Can you work these out from the model? Positions are in its coordinate system, mm. A direction names the side the tool comes from. Coordinates: 2 decimals unless noted, no trailing zeros. Order: outer loops, then holes, each group sorted by start corner. A loop starts at its lowest first (then second) coordinate and runs counter-clockwise, first axis right, second up. Notation, with made-up numbers: (14, 32.5) -> (37, 32.5) arc R18 ccw to (37, 60.5) -> close; hole circle Ø6 at (10.25, 33.25). An arc over 180 degrees is marked (long way). Write item = value, one per line. Start each with the question number.
from build123d import *
from build123d.topology import SkipClean

# Parameters (mm, degrees)
SKETCH1_R            = 22
SKETCH1_R_2          = 18
BOSS_EXTRUDE1_DEPTH  = 83
BOSS_EXTRUDE2_START  = -9
SKETCH2_R            = 18
SKETCH2_R_2          = 5.5
BOSS_EXTRUDE2_DEPTH  = 6
SKETCH6_W            = 30
SKETCH6_H            = 40
BOSS_EXTRUDE5_DEPTH  = 6
BOSS_EXTRUDE6_START  = -3
SKETCH7_R            = 12.5
SKETCH7_R_2          = 5.5
BOSS_EXTRUDE6_DEPTH  = 6
BOSS_EXTRUDE7_DEPTH  = 3
BOSS_EXTRUDE8_START  = -6
SKETCH9_R            = 12.5
SKETCH9_R_2          = 5.5
BOSS_EXTRUDE8_DEPTH  = 6
RIB1_REACH           = 137.338
SKETCH10_WALL_W      = 297.088193202
SKETCH10_WALL_H      = 6
BOSS_EXTRUDE10_DEPTH = 3
SKETCH12_R           = 12.5
SKETCH12_R_2         = 5.5
BOSS_EXTRUDE11_DEPTH = 3


with BuildPart() as part:
    # Sketch1 → Boss-Extrude1 (new body)
    with BuildSketch(Plane(origin=(0, 0, 0), x_dir=(1, 0, 0), z_dir=(0, 1, 0))):
        with Locations(Location((0, 0, 0), (0, 0, 270))):
            Circle(SKETCH1_R)
        with Locations(Location((0, 0, 0), (0, 0, 270))):
            Circle(SKETCH1_R_2, mode=Mode.SUBTRACT)
    extrude(amount=BOSS_EXTRUDE1_DEPTH)

    # Sketch2 → Boss-Extrude2 (add)
    with SkipClean():  # the faces are left unmerged after this step: merging them gives an invalid solid
        with BuildSketch(Plane(origin=(0, 83, 0), x_dir=(1, 0, 0), z_dir=(0, 1, 0)).offset(BOSS_EXTRUDE2_START)):
            with BuildLine():
                Line((-48, 20), (-48, -20))
                Line((-48, -20), (-0.924768705, -21.980555108))
                ThreePointArc((-0.924768705, -21.980555108), (1.727252911, -21.932090584), (4.354166667, -21.564814691))
                Line((4.354166667, -21.564814691), (50.473958333, -12.25273562))
                ThreePointArc((50.473958333, -12.25273562), (60.5, 0), (50.473958333, 12.25273562))
                Line((50.473958333, 12.25273562), (4.354166667, 21.564814691))
                ThreePointArc((4.354166667, 21.564814691), (1.727252911, 21.932090584), (-0.924768705, 21.980555108))
                Line((-0.924768705, 21.980555108), (-48, 20))
            make_face()
            with Locations(Location((0, 0, 0), (0, 0, 270))):
                Circle(SKETCH2_R, mode=Mode.SUBTRACT)
            with Locations(Location((48, 0, 0), (0, 0, 270))):
                Circle(SKETCH2_R_2, mode=Mode.SUBTRACT)
        extrude(amount=BOSS_EXTRUDE2_DEPTH)

    # Sketch6 → Boss-Extrude5 (add)
    with BuildSketch(Plane.ZY.offset(48)):
        with Locations((0, 77)):
            Rectangle(SKETCH6_W, SKETCH6_H)
    extrude(amount=-BOSS_EXTRUDE5_DEPTH)



with BuildPart() as body_2:
    # Sketch7 → Boss-Extrude6 (new body)
    with BuildSketch(Plane(origin=(0, 97, 0), x_dir=(1, 0, 0), z_dir=(0, 1, 0)).offset(BOSS_EXTRUDE6_START)):
        with Locations(Location((-76, 0, 0), (0, 0, 270))):
            Circle(SKETCH7_R)
        with Locations(Location((-76, 0, 0), (0, 0, 270))):
            Circle(SKETCH7_R_2, mode=Mode.SUBTRACT)
    extrude(amount=BOSS_EXTRUDE6_DEPTH)


with BuildPart() as part_1:
    add(part.part)

    add(body_2.part)  # Boss-Extrude7 merges body 2
    # Sketch8 → Boss-Extrude7 (add)
    with BuildSketch(Plane(origin=(0, 97, 0), x_dir=(1, 0, 0), z_dir=(0, 1, 0))):
        with BuildLine():
            Line((-70.062828956, 11), (-48, 11))
            Line((-48, 11), (-48, -11))
            Line((-48, -11), (-70.062828956, -11))
            ThreePointArc((-70.062828956, -11), (-63.5, 0), (-70.062828956, 11))
        make_face()
    boss_extrude7 = extrude(amount=-BOSS_EXTRUDE7_DEPTH)

    # Mirror3: Boss-Extrude7 across plane
    add(boss_extrude7.mirror(Plane.ZX.offset(77)))

    # Sketch9 → Boss-Extrude8 (add)
    with BuildSketch(Plane(origin=(0, 60, 0), x_dir=(1, 0, 0), z_dir=(0, 1, 0)).offset(BOSS_EXTRUDE8_START)):
        with Locations(Location((-76, 0, 0), (0, 0, 61.642363424))):
            Circle(SKETCH9_R)
        with Locations(Location((-76, 0, 0), (0, 0, 270))):
            Circle(SKETCH9_R_2, mode=Mode.SUBTRACT)
    extrude(amount=BOSS_EXTRUDE8_DEPTH)

    # Sketch10 wall → Rib1 (add, up to next)
    with BuildSketch(Plane(origin=(-32, 90, 0), x_dir=(0.819231920519, -0.573462344363, 0), z_dir=(0.573462344363, 0.819231920519, 0)), mode=Mode.PRIVATE) as rib1_sk1:
        Rectangle(SKETCH10_WALL_W, SKETCH10_WALL_H)
    rib1_tool1 = extrude(rib1_sk1.sketch, amount=-RIB1_REACH, mode=Mode.PRIVATE) - part_1.part
    add(rib1_tool1.solids().sort_by_distance((-32, 90, 0))[0])

    # Sketch11 → Boss-Extrude10 (add, symmetric)
    with BuildSketch(Plane.XY):
        Polygon((-42, 57), (-22, 0), (-20, 0), (-20, 74), (-42, 74), align=None)
    extrude(amount=BOSS_EXTRUDE10_DEPTH, both=True)

    # Sketch12 → Boss-Extrude11 (add)
    with BuildSketch(Plane(origin=(0, 80, 0), x_dir=(1, 0, 0), z_dir=(0, 1, 0))):
        with Locations(Location((48, 0, 0), (0, 0, 270))):
            Circle(SKETCH12_R)
        with Locations(Location((48, 0, 0), (0, 0, 270))):
            Circle(SKETCH12_R_2, mode=Mode.SUBTRACT)
    extrude(amount=BOSS_EXTRUDE11_DEPTH)


solid = part_1.part
(1) Imagine slicing it at D-D (y = 14.5). Write out the boundary of the cut face in (x, z).
(2) If I drill on L1, parallel to X at y = 67.5, z = 0; L2, parallel to X at y = 82, z = -0.5; L3, parallel to X at y = 98, z = 0, over which ranges is the centre line in solid material (lowest first)? Write a range as from..to.
(3) Thinking about a two-plate mould opening in X: for faces 5 (the face through (-30, 74, -13)), 6 (the face through (-24.133, 76.958, -21.004)), 7 (the face through (-45, 88, -15)), which applies, +X half, -X half, draft (parallel to the pull), parting line (faces both ways), or undercut?
(4) Imagine slicing it at B-B (x = -55). Write out the boundary of the cut face in (y, z), plus the area to 3 significant figures.
(5) For P1, Ø16, axis at x = -30, y = 27.5, coming from the -Z side; P2, Ø4, axis at x = 30.5, z = 15, coming from the +Y side; P3, Ø3, axis at x = -54, z = -5, coming from the -Y side, each with a flat end and sliding along its axis, tell me the tip position at first contact or that it passes through.
(6) For faces 1 (the face through (-30, 46, -3)), 2 (the face through (-59, 58, 11)), 3 (the face through (-45, 65, -15)), 4 (the face through (-45, 65, 15)), which set-ups out of +Z, -Z, +X, -X, +Y, -Y let a thin tool reach every point of the face, with its end or its side?
(7) Imagine slicing it at A-A (x = -76). Write out the boundary of the cut face in (y, z).
Result set:
q1.outline = (-27.09, -3) -> (-21.79, -3) arc R22 ccw (long way) to (-21.79, 3) -> (-27.09, 3) -> close; hole circle Ø36 at (0, 0)
q2.L1 = -48..-18, 18..22
q2.L2 = -48..-17.99, 17.99..21.99, 35.51..42.52, 53.48..60.49
q2.L3 = -88.5..-81.5, -70.5..-63.5
q3.face_5 = undercut
q3.face_6 = -X half
q3.face_7 = draft
q4.outline = (57, -11) -> (60, -11) -> (60, 11) -> (57, 11) -> close; (94, -11) -> (97, -11) -> (97, 11) -> (94, 11) -> close
q4.area = 132 mm2
q5.P1 = -3
q5.P2 = 80
q5.P3 = 57
q6.face_1 = -Z, -Y
q6.face_2 = +Z, +Y, -Y
q6.face_3 = -Z, -X, -Y
q6.face_4 = +Z, -X, -Y
q7.outline = (54, -12.5) -> (60, -12.5) -> (60, -5.5) -> (54, -5.5) -> close; (54, 5.5) -> (60, 5.5) -> (60, 12.5) -> (54, 12.5) -> close; (94, -12.5) -> (100, -12.5) -> (100, -5.5) -> (94, -5.5) -> close; (94, 5.5) -> (100, 5.5) -> (100, 12.5) -> (94, 12.5) -> close
